Build history of the part. All positions in model axes, mm. A direction names the side the tool comes from. Give positions to 0.01 mm unless a question says otherwise; leave off trailing zeros. Loops run counter-clockwise (first coordinate to the right, second up) from the corner with the lowest first, then second, coordinate; pieces in that order, holes last. Notation, with made-up numbers: M -4.75,4.25 L 17.25,4.25 A23 ccw 17.25,24.25 Z; hole C 49,39.25 d1. An arc over 180 degrees is marked long. Answer in a Markdown table with one row per item. Add a question column.
```python
from build123d import *

# Parameters (mm, degrees)
SKETCH1_R           = 63.5
BOSS_EXTRUDE1_DEPTH = 50.8
SKETCH2_R           = 25.4
CUT_EXTRUDE2_DEPTH  = 25.4
SKETCH3_R           = 6.35
CUT_EXTRUDE3_DEPTH  = 94.3255592
SKETCH6_R           = 12.7
CUT_EXTRUDE4_DEPTH  = 6.35
CHAMFER1_SIZE       = 12.7
FILLET1_R           = 6.35


with BuildPart() as part:
    # Sketch1 → Boss-Extrude1 (new body)
    with BuildSketch(Plane.XY):
        Circle(SKETCH1_R)
    extrude(amount=BOSS_EXTRUDE1_DEPTH)

    # Sketch2 → Cut-Extrude2 (cut)
    with BuildSketch(Plane.XY.offset(50.8)):
        Circle(SKETCH2_R)
    extrude(amount=-CUT_EXTRUDE2_DEPTH, mode=Mode.SUBTRACT)

    # Sketch3 → Cut-Extrude3 (cut, through all)
    with BuildSketch(Plane.XY.offset(25.4)):
        Circle(SKETCH3_R)
    extrude(amount=-CUT_EXTRUDE3_DEPTH, mode=Mode.SUBTRACT)

    # Sketch4 → Cut-Revolve1 (revolve, cut)
    with BuildSketch(Plane(origin=(0, 0, 0), x_dir=(0, 0, -1), z_dir=(1, 0, 0)), mode=Mode.PRIVATE) as cut_revolve1_sk:
        Polygon((0, 63.5), (-25.4, 63.5), (0, 6.35), align=None)
    revolve(cut_revolve1_sk.sketch.rotate(Axis((0, 0, 0), (0, 0, -1)), 90), axis=Axis((0, 0, 0), (0, 0, -1)), mode=Mode.SUBTRACT)

    # Sketch6 → Cut-Extrude4 (cut)
    with BuildSketch(Plane.XY):
        Circle(SKETCH6_R)
    extrude(amount=CUT_EXTRUDE4_DEPTH, mode=Mode.SUBTRACT)

    # Chamfer1
    chamfer1_edges = [part.edges().sort_by_distance(p)[0] for p in [
        (-63.5, 0, 50.8),
    ]]
    chamfer(chamfer1_edges, length=CHAMFER1_SIZE)

    # Fillet1
    fillet1_edges = [part.edges().sort_by_distance(p)[0] for p in [
        (-63.5, 0, 25.4),
        (-50.8, 0, 50.8),
        (-63.5, 0, 38.1),
        (-25.4, 0, 50.8),
    ]]
    fillet(fillet1_edges, radius=FILLET1_R)


solid = part.part
```
(1) Pin check, flat tips, straight feed: pin 1 (12.5 mm diameter, centred on x = -4.5, y = -3.5, fed in from -Z); pin 2 (11.5 mm diameter, centred on x = 0, y = 0, fed in from -Z) (1 decimal); pin 3 (1.5 mm diameter, centred on x = 32.5, y = 6.5, fed in from -Z); pin 4 (10 mm diameter, centred on x = -8, z = 31, fed in from +Y). Stop position of each tip, or through.
(2) Tool access for faces 4 (the cylindrical face through (-1.38, -6.2, 16.01)), 5 (the cylindrical face through (-5.506, -24.796, 35.058)), 6 (the flat face through (3, 6, 6.35)): list every direction of +Z, -Z, +X, -X, +Y, -Y with a clear straight run to the whole face (end or side of a thin tool).
(3) Pull direction X, two halves, no side cores. Call faces 1 (the flat face through (31, -10, 50.8)), 2 (the conical face through (49.05, -20.34, 48.5)), 3 (the flat face through (5, -5, 25.4)): +X half, -X half, draft (parallel to the pull), parting line (faces both ways), or undercut.
(4) Slice it at B-B, the plane z = 14. Give the cut face in (x, y), then the cut area to 3 significant figures.
(5) Wall check: line 1 (Z direction, x = -10, y = 4.5); line 2 (Y direction, x = -6, z = 49.5); line 3 (Y direction, x = 0, z = 29.5). Give the ranges that are in metal, low to high.
(6) Slice it at A-A, the plane z = 32.5. Give the cut face in (x, y).
Solution:
| question | item | result |
|---|---|---|
| 1 | pin 1 | z = 6.35 |
| 1 | pin 2 | through |
| 1 | pin 3 | z = 11.57 |
| 1 | pin 4 | y = 63.43 |
| 2 | face 4 | +Z, -Z |
| 2 | face 5 | +Z |
| 2 | face 6 | -Z |
| 3 | face 1 | draft |
| 3 | face 2 | parting line |
| 3 | face 3 | undercut |
| 4 | outline | C 0,0 d75.7; hole C 0,0 d12.7 |
| 4 | area | 4,370 mm^2 |
| 5 | line 1 | 6.35 to 25.4 |
| 5 | line 2 | -51.67 to -27.25, 27.25 to 51.67 |
| 5 | line 3 | -63.5 to -25.4, 25.4 to 63.5 |
| 6 | outline | C 0,0 d127; hole C 0,0 d50.8 |
